Autodesk Inventor part; units mm, degrees
ref_plane "YZ Plane" through (0, 0, 0) normal (1, 0, 0) x (0, 1, 0)
ref_plane "XZ Plane" through (0, 0, 0) normal (0, 1, 0) x (-1, 0, 0)
ref_plane "XY Plane" through (0, 0, 0) normal (0, 0, 1) x (1, 0, 0)
sketch "Sketch1" plane through (0, 0, 0) normal (0, 0, 1) x (1, 0, 0)
  circle A0 centre (0, 0) radius 2.5
  line L0 (1.5, 2) -> (1.5, -2)
  dimension "d0" = 5
  dimension "d1" = 1.5
extrude "Extrusion1" add sketch "Sketch1" along normal blind 90
extrude "Extrusion2" cut sketch "Sketch1" along normal blind 9 contours A0 L0 picked at (1.6398, 0.534)
chamfer "Chamfer1" distance 0.25 angle 45 2 edges at (-2.5, 0, 90) (-2.5, 0, 0)
properties part number "HeatExchangePistonShaft"
The model under review builds one solid part; all positions refer to its coordinate system, in mm. A direction names the side the tool comes from. Round coordinates to 2 decimals unless told otherwise and drop trailing zeros. Loops run counter-clockwise (first coordinate to the right, second up) from the corner with the lowest first, then second, coordinate; pieces in that order, holes last.
1) Clearance check with a flat-ended pin moving along its axis: P1, Ø3, axis at y = -0.5, z = 2.5, coming from the +X side. State where the tip first meets the part, or that it passes through.
Values follow:
P1: stops at x = 1.5
2) Wall thickness on line 1 along X through (y, z) = (-1.5, 45); line 2 along X through (y, z) = (-1.05, 11): over which ranges is each line inside the solid? List them lowest first.
Values follow:
line 1: x = -2 to 2
line 2: x = -2.27 to 2.27
3) Consider section A-A on y = 0. State the section outline as (x, z) points, then the cut area to 3 significant figures.
Values follow:
outline: (-2.5, 0.25) - (-2.25, 0) - (1.5, 0) - (1.5, 9) - (2.5, 9) - (2.5, 89.75) - (2.25, 90) - (-2.25, 90) - (-2.5, 89.75) - close
area: 441 mm2
4) Consider section B-B on z = 66. State the section outline as (x, y) points.
Values follow:
outline: circle Ø5 at (0, 0)
5) Tool access review of faces 1 (the face through (-2.38, 0.08, 0.13)), 2 (the face through (1.5, 0, 4)): name each direction out of +Z, -Z, +X, -X, +Y, -Y from which nothing blocks a thin tool from reaching the whole face with its end or side.
Values follow:
face 1: -Z
face 2: -Z, +X, +Y, -Y
